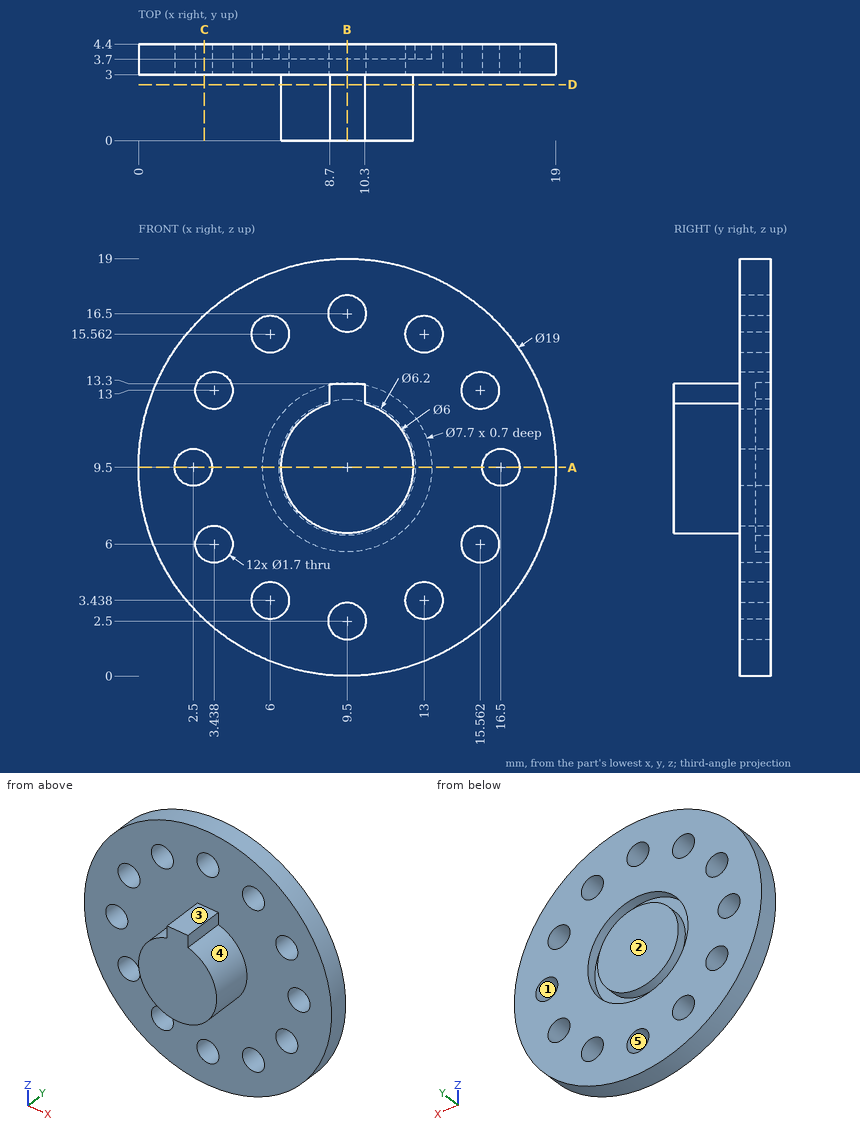
Geometry: see drawing. Coordinates: mm, zero at the bounding-box minimum. A direction names the side the tool comes from. Give positions to 0.01 mm unless a question says otherwise; leave off trailing zeros. Order: outer loops, then holes, each group sorted by start corner. A loop starts at its lowest first (then second) coordinate and runs counter-clockwise, first axis right, second up. Notation, with made-up numbers: M 47,-37 L 68,-37 A23 ccw 68,-19 Z; hole C 62.25,6 d9. An arc over 180 degrees is marked long. Answer as a JSON object with one key per item and string values.
1. Cut plane D-D, the plane y = 2.55. Output: boundary loops of the cut face in (x, z), and give its area (3 significant figures).
Result sheet:
{"outline": "M 8.7,12.39 A3 ccw long 10.3,12.39 L 10.3,13.3 L 8.7,13.3 Z", "area": "29.6 mm²"}
2. Pull-direction query (Z, two-part tool) for the marked faces 1, 2 and 3; classes: +Z half, -Z half, draft (parallel to the pull), parting line (faces both ways), or undercut.
Result sheet:
{"face 1": "undercut", "face 2": "draft", "face 3": "+Z half"}
3. First-contact query: P1, Ø1, axis at y = 1.5, z = 13.5, coming from the +X side; P2, Ø2.5, axis at x = 16.5, z = 9.5, coming from the -Y side; P3, Ø1, axis at y = 3, z = 5.5, coming from the -X side; P4, Ø1.4, axis at x = 15.56, z = 6, coming from the -Y side. Flat tips, straight axial feed; report the tip coordinate or a pass-through.
Result sheet:
{"P1": "x = 10.3", "P2": "y = 3", "P3": "x = 0.67", "P4": "through"}
4. Cut plane B-B, the plane x = 9.5. Output: boundary loops of the cut face in (y, z), and give its area (3 significant figures).
Result sheet:
{"outline": "M 0,6.5 L 3,6.5 L 3,3.35 L 4.4,3.35 L 4.4,5.65 L 3.7,5.65 L 3.7,6.4 L 4.4,6.4 L 4.4,12.6 L 3.7,12.6 L 3.7,13.35 L 4.4,13.35 L 4.4,15.65 L 3,15.65 L 3,13.3 L 0,13.3 Z; M 3,0 L 4.4,0 L 4.4,1.65 L 3,1.65 Z; M 3,17.35 L 4.4,17.35 L 4.4,19 L 3,19 Z", "area": "41.2 mm²"}
5. Ray query, line 1 (X direction, y = 4.1, z = 9.5); line 2 (X direction, y = 3.5, z = 6); line 3 (Y direction, x = 14.5, z = 17.25). Return the intervals inside material, ascending. Write a range as [from, to].
Result sheet:
{"line 1": "[0, 1.65], [3.35, 5.65], [6.4, 12.6], [13.35, 15.65], [17.35, 19]", "line 2": "[0.67, 2.59], [4.29, 14.71], [16.41, 18.33]", "line 3": "[3, 4.4]"}
6. Cut plane A-A, the plane z = 9.5. Output: boundary loops of the cut face in (x, y), and give its area (3 significant figures).
Result sheet:
{"outline": "M 0,3 L 1.65,3 L 1.65,4.4 L 0,4.4 Z; M 3.35,3 L 6.5,3 L 6.5,0 L 12.5,0 L 12.5,3 L 15.65,3 L 15.65,4.4 L 13.35,4.4 L 13.35,3.7 L 12.6,3.7 L 12.6,4.4 L 6.4,4.4 L 6.4,3.7 L 5.65,3.7 L 5.65,4.4 L 3.35,4.4 Z; M 17.35,3 L 19,3 L 19,4.4 L 17.35,4.4 Z", "area": "38.8 mm²"}
7. Cut plane C-C, the plane x = 3. Output: boundary loops of the cut face in (y, z), and give its area (3 significant figures).
Result sheet:
{"outline": "M 3,2.57 L 4.4,2.57 L 4.4,5.27 L 3,5.27 Z; M 3,6.73 L 4.4,6.73 L 4.4,8.81 L 3,8.81 Z; M 3,10.19 L 4.4,10.19 L 4.4,12.27 L 3,12.27 Z; M 3,13.73 L 4.4,13.73 L 4.4,16.43 L 3,16.43 Z", "area": "13.4 mm²"}
8. Reachability of the marked faces 4 and 5 from +Z, -Z, +X, -X, +Y, -Y: full face, straight path, thin tool, end or side. Return the list, or none.
Result sheet:
{"face 4": "-Y", "face 5": "+Y, -Y"}
